Geometry: see drawing. Coordinates: mm, zero at the bounding-box minimum. A direction names the side the tool comes from. Coordinates: 2 decimals unless noted, no trailing zeros. Write each loop counter-clockwise with the first axis right and the second up, starting at its lowest first coordinate (ties: lowest second). Pieces come first, ordered by that corner, then holes.
1) Pin query (flat end, axial travel): pin 1 Ø5.5 at (x, y) = (60, 8.5) entering from +Z; pin 2 Ø5 at (y, z) = (5, 45.5) entering from +X. Return the tip coordinate at first contact, or that it passes through.
2) Section query B-B (z = 40). Output: boundary loops of the cut face in (x, y).
3) Section query D-D (z = 21). Output: boundary loops of the cut face in (x, y).
4) Set-up query: the marked faces 4 and 5. Return all of +Z, -Z, +X, -X, +Y, -Y with unobstructed straight access to the full face (end or side cutting, diameter ignored); none if empty.
5) Section query A-A (x = 49). Output: boundary loops of the cut face in (y, z) (1 decimal).
6) Line query: L1, parallel to X at y = 3.5, z = 45.5; L2, parallel to Z at x = 64, y = 15.25; L3, parallel to X at y = 13, z = 36.5. Output: solid intervals per line, ascending.
7) Draft query along X for the marked faces 1, 2 and 3. Return one class per face: pulls with the +X half, pulls with the -X half, needs draft (parallel to the pull), parting line crosses it, or undercut.
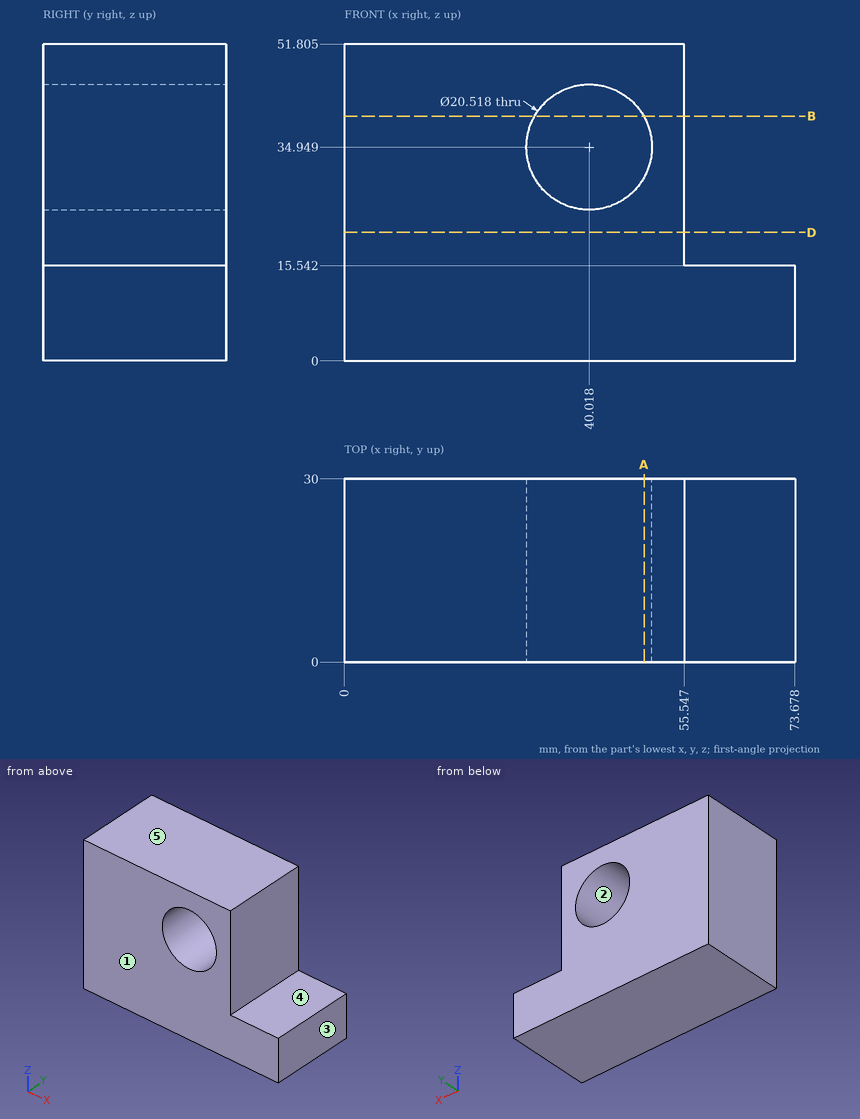
Answer:
1. pin 1: stops at z = 15.54
1. pin 2: stops at x = 55.55
2. outline: (0, 0) - (31.09, 0) - (31.09, 30) - (0, 30) - close; (48.95, 0) - (55.55, 0) - (55.55, 30) - (48.95, 30) - close
3. outline: (0, 0) - (55.55, 0) - (55.55, 30) - (0, 30) - close
4. face 4: +Z, +X, +Y, -Y
4. face 5: +Z, +X, -X, +Y, -Y
5. outline: (0, 0) - (30, 0) - (30, 30) - (0, 30) - close; (0, 39.9) - (30, 39.9) - (30, 51.8) - (0, 51.8) - close
6. L1: x = 0 to 55.55
6. L2: z = 0 to 15.54
6. L3: x = 0 to 29.88, 50.16 to 55.55
7. face 1: needs draft
7. face 2: undercut
7. face 3: pulls with the +X half
